```python
from build123d import *

# Parameters (mm, degrees)
ESBO_O1_W                = 26.6
ESBO_O1_H                = 13.3
RESSALTO_EXTRUS_O1_DEPTH = 10
ESBO_O2_R                = 1.75
CORTE_EXTRUS_O1_DEPTH    = 18.919612776
ESBO_O3_R                = 8.48
CORTE_EXTRUS_O2_DEPTH    = 4.3
ESBO_O3_3_R              = 6.25
CORTE_EXTRUS_O3_DEPTH    = 9.8
CORTE_EXTRUS_O4_START    = -3.5
ESBO_O4_R                = 8.48
CORTE_EXTRUS_O4_DEPTH    = 3.5
RESSALTO_EXTRUS_O2_START = -13.3
RESSALTO_EXTRUS_O2_DEPTH = 13.3
RESSALTO_EXTRUS_O3_DEPTH = 5.5
ESBO_O7_W                = 1.347129382
ESBO_O7_H                = 0.427620669
RESSALTO_EXTRUS_O4_DEPTH = 5.5


with BuildPart() as part:
    # Esboço1 → Ressalto-extrusão1 (new body)
    with BuildSketch(Plane(origin=(7.1e-08, 2.4e-08, -1.999994237), x_dir=(-0.9999999999999994, 0, -3.5493490277080375e-08), z_dir=(3.5493490277080375e-08, 1.1940033902129589e-08, -0.9999999999999994))):
        Rectangle(ESBO_O1_W, ESBO_O1_H)
    extrude(amount=-RESSALTO_EXTRUS_O1_DEPTH)

    # Esboço2 → Corte-extrusão1 (cut, through all)
    with BuildSketch(Plane(origin=(7.1e-08, 2.4e-08, -1.999994237), x_dir=(-0.9999999999999994, 0, -3.549349026814977e-08), z_dir=(3.5493490268149776e-08, 1.1940033893980961e-08, -0.9999999999999994))):
        with Locations((-10.5, 0)):
            Circle(ESBO_O2_R)
        with Locations(Location((10.5, 0, 0), (0, 0, 180))):
            Circle(ESBO_O2_R)
    extrude(amount=-CORTE_EXTRUS_O1_DEPTH, mode=Mode.SUBTRACT)

    # Esboço3 → Corte-extrusão2 (cut)
    with BuildSketch(Plane(origin=(0, 6.65, 7.9e-08), x_dir=(1, 0, 0), z_dir=(0, 1.0, 1.1940033902129584e-08))):
        with Locations((0, -12.300005763)):
            Circle(ESBO_O3_R)
    extrude(amount=-CORTE_EXTRUS_O2_DEPTH, mode=Mode.SUBTRACT)

    # Esboço3<3> → Corte-extrusão3 (cut)
    with BuildSketch(Plane(origin=(0, 6.65, 7.9e-08), x_dir=(1, 0, 0), z_dir=(0, 1.0, 1.1940033902129584e-08))):
        with Locations((0, -12.300005763)):
            Circle(ESBO_O3_3_R)
    extrude(amount=-CORTE_EXTRUS_O3_DEPTH, mode=Mode.SUBTRACT)

    # Esboço4 → Corte-extrusão4 (cut)
    with BuildSketch(Plane(origin=(0, -6.65, -7.9e-08), x_dir=(1, 0, 0), z_dir=(0, -1.0, -1.1940033902129595e-08)).offset(CORTE_EXTRUS_O4_START)):
        with Locations((0, 12.300005763)):
            Circle(ESBO_O4_R)
    extrude(amount=CORTE_EXTRUS_O4_DEPTH, mode=Mode.SUBTRACT)

    # Esboço5 → Ressalto-extrusão2 (add)
    with BuildSketch(Plane(origin=(0, 6.65, 7.9e-08), x_dir=(1, 0, 0), z_dir=(0, 1.0, 1.1940033902129584e-08)).offset(RESSALTO_EXTRUS_O2_START)):
        Polygon((-7.249600207, -7.90072209), (-3.073568805, -4.39661568), (-6.960916747, -4.39661568), align=None)
        Polygon((7.249600207, -7.90072209), (3.073568805, -4.39661568), (6.960916747, -4.39661568), align=None)
        Polygon((-2.666064515, -4.250005763), (2.666064515, -4.250005763), (0, -3.025002882), align=None)
    extrude(amount=RESSALTO_EXTRUS_O2_DEPTH)

    # Esboço6 → Ressalto-extrusão3 (add)
    with BuildSketch(Plane(origin=(0, 2.35, 2.8e-08), x_dir=(1, 0, 0), z_dir=(0, 1.0, 1.1940033914348732e-08))):
        Polygon((-4.561360471, -8.027244285), (-1.243296754, -6.480005763), (1.243296754, -6.480005763), (4.561360471, -8.027244285), (3.582423284, -5.971627344), (0.394906827, -6.062494352), (-0.394906827, -6.062494352), (-3.582423284, -5.971627344), align=None)
    extrude(amount=-RESSALTO_EXTRUS_O3_DEPTH)

    # Esboço7 → Ressalto-extrusão4 (add)
    with BuildSketch(Plane(origin=(0, 2.35, 2.8e-08), x_dir=(1, 0, 0), z_dir=(0, 1.0, 1.1940033894814705e-08))):
        with Locations((0, -6.062494352)):
            Rectangle(ESBO_O7_W, ESBO_O7_H)
    extrude(amount=-RESSALTO_EXTRUS_O4_DEPTH)


solid = part.part
```
Design review of the part built by this model. Coordinates are the model's own, in mm. A direction names the side the tool comes from. Give positions to 0.01 mm unless a question says otherwise; leave off trailing zeros. Write each loop counter-clockwise with the first axis right and the second up, starting at its lowest first coordinate (ties: lowest second). Pieces come first, ordered by that corner, then holes. Notation, with made-up numbers: (66.25, 12) - (93.25, 12) arc R9 ccw to (93.25, 18) - close; hole circle Ø7 at (42.25, 40.5). An arc over 180 degrees is marked (long way). Return JSON: item names as keys, results as strings. Group by question number.
(1) Insertion check: pin 1 (4.5 mm diameter, centred on x = 1, y = 4, fed in from +Z); pin 2 (2 mm diameter, centred on x = -4, y = 1, fed in from +Z); pin 3 (2 mm diameter, centred on x = -10.5, y = 0, fed in from -Z); pin 4 (1.9 mm diameter, centred on x = 3.5, z = 6.5, fed in from +Y). Each pin has a flat end and moves straight along its axis. Give the tip position at first contact, or say it passes through.
(2) To check wall thickness, follow probe 1 along X at (y, z) = (0, 6); probe 2 along Y at (x, z) = (-10.5, 3). State the ranges of each line that lie inside material, in increasing order.
(3) Machinability: for faces 4 (the flat face through (-2.926, -0.362, 7.264)), 5 (the flat face through (0, -5, 4.25)), 6 (the flat face through (0, 0, -2)), 7 (the flat face through (0, 2.35, 6)), which of the approach directions +Z, -Z, +X, -X, +Y, -Y give a long, thin tool a straight path to every point of the face, cutting with its end or side? Answer none if there is none.
(4) We need section A-A, the plane y = 0. Give the number of separate pieces and of enclosed holes in the cut face, then the cut area to 3 significant figures.
(5) Mouldability with a two-part tool opening along X and no side actions: class faces 1 (the flat face through (-8.9, -1.4, 8)), 2 (the flat face through (0, -3.15, 6)), 3 (the flat face through (-13.3, 0, 3)) as +X half, -X half, draft (parallel to the pull), parting line (faces both ways), or undercut.
(6) We need section B-B, the plane z = -0.75. Give the boundary of the cut face in (x, y), then the cut area to 3 significant figures.
Reported:
{
 "1": {"pin 1": "stops at z = 7.08", "pin 2": "stops at z = 8.03", "pin 3": "passes through", "pin 4": "stops at y = 2.35"},
 "2": {"probe 1": "x = -13.3 to -12.25, -8.75 to 8.75, 12.25 to 13.3", "probe 2": "y = -6.65 to -1.75, 1.75 to 6.65"},
 "3": {"face 4": "+Z, +Y, -Y", "face 5": "+Z, -Y", "face 6": "-Z, +X, -X, +Y, -Y", "face 7": "+Z, +Y"},
 "4": {"separate pieces": "3", "enclosed holes": "0", "area": "187 mm2"},
 "5": {"face 1": "draft", "face 2": "undercut", "face 3": "-X half"},
 "6": {"outline": "(-13.3, -6.65) - (13.3, -6.65) - (13.3, 6.65) - (-13.3, 6.65) - close; hole circle Ø3.5 at (-10.5, 0); hole circle Ø3.5 at (10.5, 0)", "area": "335 mm2"}
}
